Check sheet for the drawn part. Datum: minimum x, y, z corner. Units: mm. A direction names the side the tool comes from. Coordinates: 2 decimals unless noted, no trailing zeros. Loops run counter-clockwise (first coordinate to the right, second up) from the corner with the lowest first, then second, coordinate; pieces in that order, holes last. Notation, with made-up numbers: (13, -6.75) - (72, -6.75) arc R4 cw to (72, 0.25) - close; hole circle Ø5 at (-31, 75.5). An arc over 180 degrees is marked (long way). Answer as a JSON object with one key per item and string values. Group by question number.
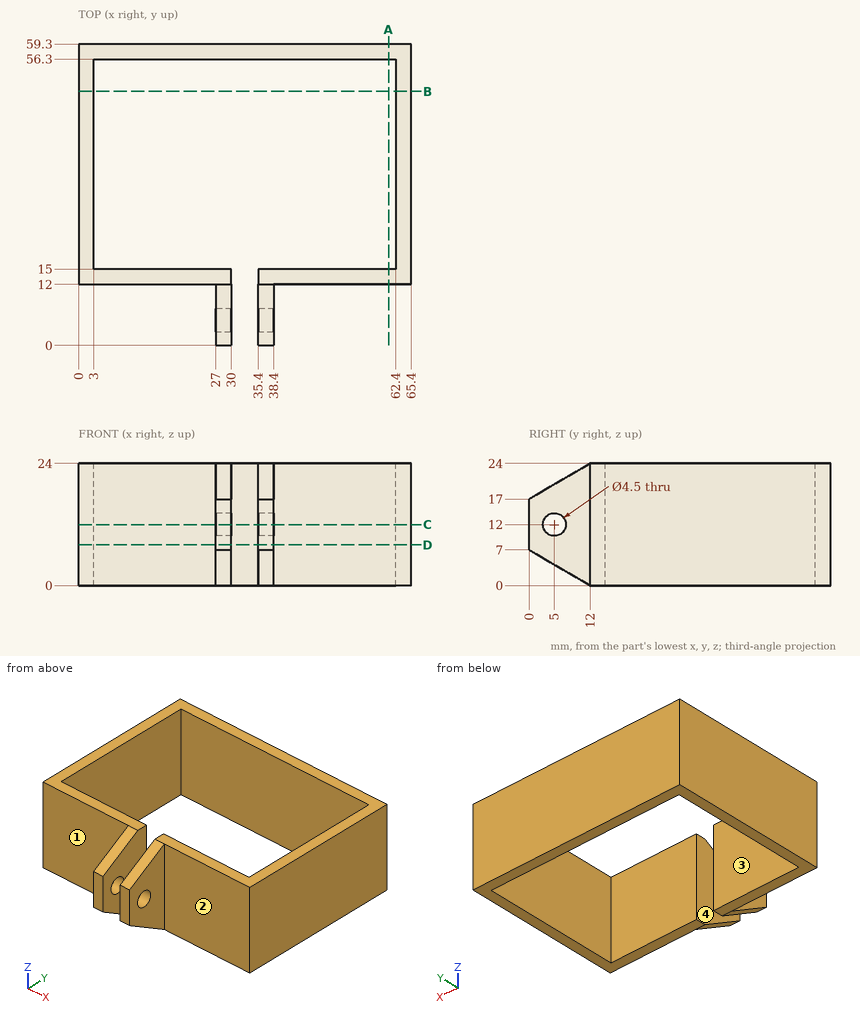
1. Gauge pin test, flat ends, axial feed: pin 1 (8 mm diameter, centred on x = 7, z = 17, fed in from -Y); pin 2 (4 mm diameter, centred on x = 38, y = 7.5, fed in from +Z); pin 3 (6 mm diameter, centred on y = 5, z = 12, fed in from +X); pin 4 (3 mm diameter, centred on x = 7.5, y = 53.5, fed in from -Z). Record the tip position at first contact, or that the pin passes through.
2. Access from +Z, -Z, +X, -X, +Y, -Y to the whole of each face (thin tool, end or side, straight path). Record for the marked faces 1, 2, 3 and 4.
3. Sectioned sample at C-C on z = 12. Record the cut outline in (x, y), plus the area to 3 significant figures.
4. Material ranges on line 1 (X direction, y = 45, z = 17); line 2 (Y direction, x = 57, z = 2.5); line 3 (X direction, y = 14, z = 5.5), recorded low to high.
5. Sectioned sample at A-A on x = 61. Record the cut outline in (y, z).
6. Sectioned sample at B-B on y = 50. Record the cut outline in (x, z), plus the area to 3 significant figures.
7. Sectioned sample at D-D on z = 8. Record the cut outline in (x, y), plus the area to 3 significant figures.
Answers follow:
{
 "1": {"pin 1": "stops at y = 12", "pin 2": "stops at z = 22.54", "pin 3": "stops at x = 38.4", "pin 4": "passes through"},
 "2": {"face 1": "+Z, -Z, -X, -Y", "face 2": "+Z, -Z, +X, -Y", "face 3": "+Z, -Z", "face 4": "+Z, -Z, -Y"},
 "3": {"outline": "(0, 12) - (27, 12) - (27, 7.25) - (30, 7.25) - (30, 15) - (3, 15) - (3, 56.3) - (62.4, 56.3) - (62.4, 15) - (35.4, 15) - (35.4, 7.25) - (38.4, 7.25) - (38.4, 12) - (65.4, 12) - (65.4, 59.3) - (0, 59.3) - close; (27, 0) - (30, 0) - (30, 2.75) - (27, 2.75) - close; (35.4, 0) - (38.4, 0) - (38.4, 2.75) - (35.4, 2.75) - close", "area": "669 mm^2"},
 "4": {"line 1": "x = 0 to 3, 62.4 to 65.4", "line 2": "y = 12 to 15, 56.3 to 59.3", "line 3": "x = 0 to 30, 35.4 to 65.4"},
 "5": {"outline": "(12, 0) - (15, 0) - (15, 24) - (12, 24) - close; (56.3, 0) - (59.3, 0) - (59.3, 24) - (56.3, 24) - close"},
 "6": {"outline": "(0, 0) - (3, 0) - (3, 24) - (0, 24) - close; (62.4, 0) - (65.4, 0) - (65.4, 24) - (62.4, 24) - close", "area": "144 mm^2"},
 "7": {"outline": "(0, 12) - (27, 12) - (27, 0) - (30, 0) - (30, 15) - (3, 15) - (3, 56.3) - (62.4, 56.3) - (62.4, 15) - (35.4, 15) - (35.4, 0) - (38.4, 0) - (38.4, 12) - (65.4, 12) - (65.4, 59.3) - (0, 59.3) - close", "area": "696 mm^2"}
}
